Could you check a few things on this model? Use its own coordinates, in mm. Give positions to 0.01 mm unless a question says otherwise; leave off trailing zeros. Loops run counter-clockwise (first coordinate to the right, second up) from the corner with the lowest first, then second, coordinate; pieces in that order, holes last. Notation, with made-up numbers: M 62.25,82 L 118.25,82 A20 ccw 118.25,93 Z; hole C 34,44 d7. An arc over 180 degrees is marked long. Answer in a Markdown table with one row per item. Add a question column.
1. If we section it at C-C on x = 5: List the corners of the cut face in (y, z) for me, then the cut area to 3 significant figures.
2. If we section it at A-A on y = 5: List the corners of the cut face in (x, z) for me, then the cut area to 3 significant figures.
3. If we section it at B-B on y = -28.15: List the corners of the cut face in (x, z) for me.
4. If we section it at D-D on z = 0.3: Count the separate pieces of the cut face and the enclosed holes in it, then the cut area to 3 significant figures.
5. I need wall thicknesses on line 1 along Y through (x, z) = (16, 1.2); line 2 along X through (y, z) = (6.5, 1.5); line 3 along Y through (x, z) = (-16, 0.8). Which ranges of each line are inside material? Lowest first, please. Write a range as from..to.
6. I'm going to push flat-ended pins straight in: pin 1 Ø1.8 at (x, y) = (-16.7, -28.15) entering from +Z; pin 2 Ø0.6 at (x, z) = (-7, 1.5) entering from +Y; pin 3 Ø1 at (y, z) = (-21, 1) entering from -X; pin 4 Ø1 at (y, z) = (18.5, 1) entering from +X. Where does each tip first touch, or does it pass through?
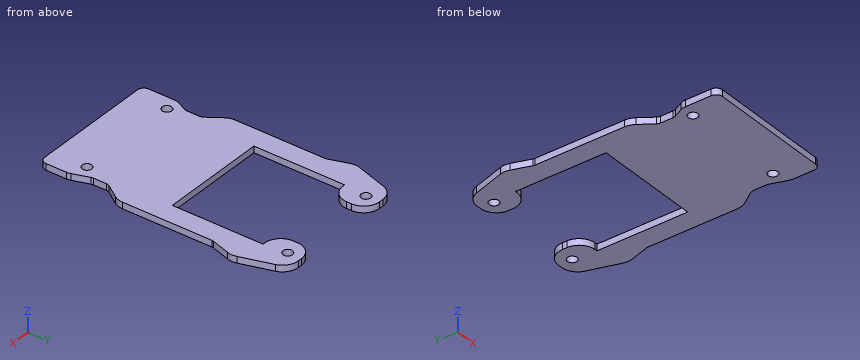
```python
from build123d import *

# Parameters (mm, degrees)
F0_R     = 1.5
F1_DEPTH = 2
F2_R     = 5
F3_R     = 2
F4_R     = 4


with BuildPart() as f1:
    # F0 (on Top) → F1 (new body)
    with BuildSketch(Plane.XY):
        Polygon((16.7, -0.85), (-16.7, -0.85), (-16.7, 27.65), (-11, 27.65), (-11, 39.15), (-21, 39.15), (-25.6, 24.35), (-23.1, 16.824023), (-23.1, -13.15), (-19, -19.15), (-19, -24.15), (-21, -28.15), (-21, -39.15), (21, -39.15), (21, -30.170781), (19, -24.15), (19, -19.15), (23.1, -13.15), (23.1, 16.824023), (25.439155, 24.35), (21, 39.15), (11, 39.15), (11, 27.65), (16.7, 27.65), align=None)
        with Locations((-16.7, -28.15)):
            Circle(F0_R, mode=Mode.SUBTRACT)
        with Locations((16, -28.15)):
            Circle(F0_R, mode=Mode.SUBTRACT)
        with Locations((-16, 34.85)):
            Circle(F0_R, mode=Mode.SUBTRACT)
        with Locations((16, 34.85)):
            Circle(F0_R, mode=Mode.SUBTRACT)
    extrude(amount=F1_DEPTH)

    # F2
    f2_edges = [f1.edges().sort_by_distance(p)[0] for p in [
        (-11, 27.65, 1),
        (11, 27.65, 1),
        (11, 39.15, 1),
        (21, 39.15, 1),
        (-11, 39.15, 1),
        (-21, 39.15, 1),
        (-25.6, 24.35, 1),
        (25.439155, 24.35, 1),
        (23.1, -13.15, 1),
        (-23.1, -13.15, 1),
    ]]
    fillet(f2_edges, radius=F2_R)

    # F3
    f3_edges = [f1.edges().sort_by_distance(p)[0] for p in [
        (23.1, 16.824023, 1),
        (-23.1, 16.824023, 1),
        (-19, -19.15, 1),
        (-19, -24.15, 1),
        (19, -19.15, 1),
        (19, -24.15, 1),
        (21, -39.15, 1),
        (-21, -39.15, 1),
    ]]
    fillet(f3_edges, radius=F3_R)

    # F4
    f4_edges = [f1.edges().sort_by_distance(p)[0] for p in [
        (-21, -28.15, 1),
        (21, -30.170781, 1),
    ]]
    fillet(f4_edges, radius=F4_R)


solid = f1.part
```
Results:
| question | item | result |
|---|---|---|
| 1 | outline | M -39.15,0 L -0.85,0 L -0.85,2 L -39.15,2 Z |
| 1 | area | 76.6 mm2 |
| 2 | outline | M -23.1,0 L -16.7,0 L -16.7,2 L -23.1,2 Z; M 16.7,0 L 23.1,0 L 23.1,2 L 16.7,2 Z |
| 2 | area | 25.6 mm2 |
| 3 | outline | M -20.89,0 L -18.2,0 L -18.2,2 L -20.89,2 Z; M -15.2,0 L 14.5,0 L 14.5,2 L -15.2,2 Z; M 17.5,0 L 20.33,0 L 20.33,2 L 17.5,2 Z |
| 4 | separate pieces | 1 |
| 4 | enclosed holes | 4 |
| 4 | area | 2,240 mm2 |
| 5 | line 1 | -39.15..-29.65, -26.65..-0.85, 27.65..33.35, 36.35..39.15 |
| 5 | line 2 | -23.1..-16.7, 16.7..23.1 |
| 5 | line 3 | -39.15..-29.48, -26.82..-0.85, 27.65..33.35, 36.35..39.15 |
| 6 | pin 1 | through |
| 6 | pin 2 | y = -0.85 |
| 6 | pin 3 | x = -19 |
| 6 | pin 4 | x = 23.78 |
